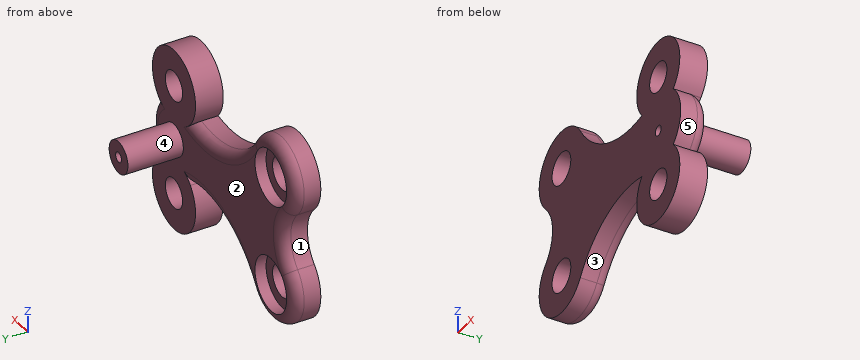
```python
from build123d import *

# Parameters (mm, degrees)
CROQUIS2_R              = 1.45
CROQUIS2_R_2            = 1.335493539
SALIENTE_EXTRUIR1_DEPTH = 2.5
CROQUIS3_R              = 2.45
CORTAR_EXTRUIR1_DEPTH   = 1
CROQUIS4_R              = 1.45
CROQUIS4_R_2            = 0.45
SALIENTE_EXTRUIR2_DEPTH = 5
CROQUIS5_R              = 0.45
CORTAR_EXTRUIR2_DEPTH   = 21.921953183
REDONDEO1_R             = 1


with BuildPart() as part:
    # Croquis2 → Saliente-Extruir1 (new body)
    with BuildSketch(Plane(origin=(0, 0, 0), x_dir=(1, 0, 0), z_dir=(0, 1, 0))):
        with BuildLine():
            ThreePointArc((17.31117806, -2.595010785), (18.475, 0), (17.31117806, 2.595010785))
            ThreePointArc((17.31117806, 2.595010785), (15.166848951, 8.331317844), (12.46008331, 2.837977715))
            ThreePointArc((12.46008331, 2.837977715), (7.057861128, 3.344392229), (2.913938348, 6.8470147))
            ThreePointArc((2.913938348, 6.8470147), (-2.156353419, 7.693072582), (-2.439518395, 2.560481605))
            ThreePointArc((-2.439518395, 2.560481605), (-1.378932188, 0), (-2.439518395, -2.560481605))
            ThreePointArc((-2.439518395, -2.560481605), (-2.156353419, -7.693072582), (2.913938348, -6.8470147))
            ThreePointArc((2.913938348, -6.8470147), (7.057861128, -3.344392229), (12.46008331, -2.837977715))
            ThreePointArc((12.46008331, -2.837977715), (15.166848951, -8.331317844), (17.31117806, -2.595010785))
        make_face()
        with Locations(Location((0, 5, 0), (0, 0, 270))):
            Circle(CROQUIS2_R, mode=Mode.SUBTRACT)
        with Locations(Location((0, -5, 0), (0, 0, 90))):
            Circle(CROQUIS2_R, mode=Mode.SUBTRACT)
        with Locations(Location((15, -5, 0), (0, 0, 270))):
            Circle(CROQUIS2_R_2, mode=Mode.SUBTRACT)
        with Locations(Location((15, 5, 0), (0, 0, 90))):
            Circle(CROQUIS2_R_2, mode=Mode.SUBTRACT)
    extrude(amount=SALIENTE_EXTRUIR1_DEPTH)

    # Croquis3 → Cortar-Extruir1 (cut)
    with BuildSketch(Plane(origin=(0, 2.5, 0), x_dir=(1, 0, 0), z_dir=(0, 1, 0))):
        with Locations(Location((0, 5, 0), (0, 0, 270))):
            Circle(CROQUIS3_R)
        with Locations(Location((0, -5, 0), (0, 0, 270))):
            Circle(CROQUIS3_R)
    extrude(amount=-CORTAR_EXTRUIR1_DEPTH, mode=Mode.SUBTRACT)

    # Croquis4 → Saliente-Extruir2 (add)
    with BuildSketch(Plane(origin=(0, 2.5, 0), x_dir=(1, 0, 0), z_dir=(0, 1, 0))):
        with Locations(Location((15, 0, 0), (0, 0, 270))):
            Circle(CROQUIS4_R)
        with Locations(Location((15, 0, 0), (0, 0, 270))):
            Circle(CROQUIS4_R_2, mode=Mode.SUBTRACT)
    extrude(amount=SALIENTE_EXTRUIR2_DEPTH)

    # Croquis5 → Cortar-Extruir2 (cut, through all)
    with BuildSketch(Plane(origin=(0, 2.5, 0), x_dir=(1, 0, 0), z_dir=(0, 1, 0))):
        with Locations(Location((15, 0, 0), (0, 0, 270))):
            Circle(CROQUIS5_R)
    extrude(amount=-CORTAR_EXTRUIR2_DEPTH, mode=Mode.SUBTRACT)

    # Redondeo1
    # the kernel refuses this fillet: 1 mm, written as the material it takes off along each edge
    with BuildSketch(Plane(origin=(10.565709674, 2.5, 11.697129023), x_dir=(-0.8446198111127597, 0, -0.5353665797151015), z_dir=(-0.5353665797151015, 0, 0.8446198111127597))) as redondeo1_piece_1_section:
        with BuildLine():
            CenterArc((9.059426769 + REDONDEO1_R, REDONDEO1_R), REDONDEO1_R, 180, 90)
            Line((9.059426769, REDONDEO1_R), (9.059426769 - REDONDEO1_R * 0.02, REDONDEO1_R))
            Line((9.059426769 - REDONDEO1_R * 0.02, REDONDEO1_R), (9.059426769 - REDONDEO1_R * 0.02, -REDONDEO1_R * 0.02))
            Line((9.059426769 - REDONDEO1_R * 0.02, -REDONDEO1_R * 0.02), (9.059426769 + REDONDEO1_R, -REDONDEO1_R * 0.02))
            Line((9.059426769 + REDONDEO1_R, -REDONDEO1_R * 0.02), (9.059426769 + REDONDEO1_R, 0))
        make_face()
    redondeo1_piece_1 = revolve(axis=Axis((10.565709674, 2.5, 11.697129023), (0, -1, 0)), revolution_arc=85.516050129, mode=Mode.PRIVATE)
    redondeo1_piece_1 = redondeo1_piece_1 - Plane(origin=(15, 2.217210624, 5), x_dir=(-0.7614815197926343, 0, -0.6481866205147249), z_dir=(0, -1, 0)) * Cylinder(3.335493539, 41, mode=Mode.PRIVATE)
    add(redondeo1_piece_1, mode=Mode.SUBTRACT)
    with BuildSketch(Plane(origin=(15, 2.5, 0), x_dir=(0.007852951460832107, 0, 0.9999691651012815), z_dir=(-0.9999691651012815, 0, 0.007852951460832107))) as redondeo1_piece_2_section:
        with BuildLine():
            CenterArc((3.475 - REDONDEO1_R, -REDONDEO1_R), REDONDEO1_R, 0, 90)
            Line((3.475, -REDONDEO1_R), (3.475 + REDONDEO1_R * 0.02, -REDONDEO1_R))
            Line((3.475 + REDONDEO1_R * 0.02, -REDONDEO1_R), (3.475 + REDONDEO1_R * 0.02, REDONDEO1_R * 0.02))
            Line((3.475 + REDONDEO1_R * 0.02, REDONDEO1_R * 0.02), (3.475 - REDONDEO1_R, REDONDEO1_R * 0.02))
            Line((3.475 - REDONDEO1_R, REDONDEO1_R * 0.02), (3.475 - REDONDEO1_R, 0))
        make_face()
    redondeo1_piece_2 = revolve(axis=Axis((15, 2.5, 0), (0, 1, 0)), revolution_arc=179.1001088, mode=Mode.PRIVATE)
    redondeo1_piece_2 = redondeo1_piece_2 - Plane(origin=(15, 2.215042964, -5), x_dir=(0.6929043732212018, 0, 0.7210294928579091), z_dir=(0, -1, 0)) * Cylinder(3.335493539, 14, mode=Mode.PRIVATE)
    redondeo1_piece_2 = redondeo1_piece_2 - Plane(origin=(15, 2.215042964, 5), x_dir=(-0.7614815197926343, 0, -0.6481866205147249), z_dir=(0, -1, 0)) * Cylinder(3.335493539, 14, mode=Mode.PRIVATE)
    add(redondeo1_piece_2, mode=Mode.SUBTRACT)
    with BuildSketch(Plane(origin=(10.565709674, 2.5, -11.697129023), x_dir=(0.4676957368071937, 0, 0.883889528036381), z_dir=(0.883889528036381, 0, -0.4676957368071937))) as redondeo1_piece_3_section:
        with BuildLine():
            CenterArc((9.059426769 + REDONDEO1_R, REDONDEO1_R), REDONDEO1_R, 180, 90)
            Line((9.059426769 + REDONDEO1_R, 0), (9.059426769 + REDONDEO1_R, -REDONDEO1_R * 0.02))
            Line((9.059426769 + REDONDEO1_R, -REDONDEO1_R * 0.02), (9.059426769 - REDONDEO1_R * 0.02, -REDONDEO1_R * 0.02))
            Line((9.059426769 - REDONDEO1_R * 0.02, -REDONDEO1_R * 0.02), (9.059426769 - REDONDEO1_R * 0.02, REDONDEO1_R))
            Line((9.059426769 - REDONDEO1_R * 0.02, REDONDEO1_R), (9.059426769, REDONDEO1_R))
        make_face()
    redondeo1_piece_3 = revolve(axis=Axis((10.565709674, 2.5, -11.697129023), (0, -1, 0)), revolution_arc=85.516050129, mode=Mode.PRIVATE)
    redondeo1_piece_3 = redondeo1_piece_3 - Plane(origin=(15, 2.217210619, -5), x_dir=(0.6929043732212018, 0, 0.7210294928579091), z_dir=(0, -1, 0)) * Cylinder(3.335493539, 41, mode=Mode.PRIVATE)
    add(redondeo1_piece_3, mode=Mode.SUBTRACT)
    with BuildSketch(Plane(origin=(0, 2.5, -5), x_dir=(0.8446198111127605, 0, -0.5353665797151004), z_dir=(0.5353665797151004, 0, 0.8446198111127605))) as redondeo1_piece_4:
        with BuildLine():
            CenterArc((3.45 - REDONDEO1_R, -REDONDEO1_R), REDONDEO1_R, 0, 90)
            Line((3.45 - REDONDEO1_R, 0), (3.45 - REDONDEO1_R, REDONDEO1_R * 0.02))
            Line((3.45 - REDONDEO1_R, REDONDEO1_R * 0.02), (3.45 + REDONDEO1_R * 0.02, REDONDEO1_R * 0.02))
            Line((3.45 + REDONDEO1_R * 0.02, REDONDEO1_R * 0.02), (3.45 + REDONDEO1_R * 0.02, -REDONDEO1_R))
            Line((3.45 + REDONDEO1_R * 0.02, -REDONDEO1_R), (3.45, -REDONDEO1_R))
        make_face()
    revolve(axis=Axis((0, 2.5, -5), (0, 1, 0)), revolution_arc=192.631224639, mode=Mode.SUBTRACT)
    with BuildSketch(Plane(origin=(-5, 2.5, 0), x_dir=(0.7071067811865475, 0, -0.7071067811865476), z_dir=(-0.7071067811865476, 0, -0.7071067811865475))) as redondeo1_piece_5:
        with BuildLine():
            CenterArc((3.621067812 + REDONDEO1_R, REDONDEO1_R), REDONDEO1_R, 180, 90)
            Line((3.621067812 + REDONDEO1_R, 0), (3.621067812 + REDONDEO1_R, -REDONDEO1_R * 0.02))
            Line((3.621067812 + REDONDEO1_R, -REDONDEO1_R * 0.02), (3.621067812 - REDONDEO1_R * 0.02, -REDONDEO1_R * 0.02))
            Line((3.621067812 - REDONDEO1_R * 0.02, -REDONDEO1_R * 0.02), (3.621067812 - REDONDEO1_R * 0.02, REDONDEO1_R))
            Line((3.621067812 - REDONDEO1_R * 0.02, REDONDEO1_R), (3.621067812, REDONDEO1_R))
        make_face()
    revolve(axis=Axis((-5, 2.5, 0), (0, -1, 0)), revolution_arc=90, mode=Mode.SUBTRACT)
    with BuildSketch(Plane(origin=(0, 2.5, 5), x_dir=(-0.7071067811865475, 0, -0.7071067811865476), z_dir=(0.7071067811865476, 0, -0.7071067811865475))) as redondeo1_piece_6:
        with BuildLine():
            CenterArc((3.45 - REDONDEO1_R, -REDONDEO1_R), REDONDEO1_R, 0, 90)
            Line((3.45, -REDONDEO1_R), (3.45 + REDONDEO1_R * 0.02, -REDONDEO1_R))
            Line((3.45 + REDONDEO1_R * 0.02, -REDONDEO1_R), (3.45 + REDONDEO1_R * 0.02, REDONDEO1_R * 0.02))
            Line((3.45 + REDONDEO1_R * 0.02, REDONDEO1_R * 0.02), (3.45 - REDONDEO1_R, REDONDEO1_R * 0.02))
            Line((3.45 - REDONDEO1_R, REDONDEO1_R * 0.02), (3.45 - REDONDEO1_R, 0))
        make_face()
    revolve(axis=Axis((0, 2.5, 5), (0, 1, 0)), revolution_arc=192.631224639, mode=Mode.SUBTRACT)


solid = part.part
```
CAD build for the part. Positions are in the model's coordinates, mm. Face numbers are marked on the shaded views. A direction names the side the tool comes from. Give positions to 0.01 mm unless a question says otherwise; leave off trailing zeros. Write each loop counter-clockwise with the first axis right and the second up, starting at its lowest first coordinate (ties: lowest second). Pieces come first, ordered by that corner, then holes. Notation, with made-up numbers: M 43,89.25 L 62,89.25 A25 ccw 62,118.25 Z; hole C 59,-10.5 d4. An arc over 180 degrees is marked long. Return JSON: item names as keys, results as strings. Group by question number.
(1) Band-saw the part on C-C (x = 0). Give the cut face in (y, z), and give its area (3 significant figures).
(2) Band-saw the part on D-D (y = 2.25). Give the cut face in (x, z).
(3) Mould opens along X. For the marked faces 1, 2 and 3 say: pulls with the +X half, pulls with the -X half, needs draft (parallel to the pull), parting line crosses it, or undercut.
(4) 3-axis set-ups, long thin cutter, end or side, ignore diameter. For the marked faces 4 and 5: which of +Z, -Z, +X, -X, +Y, -Y reach the whole face in a straight line?
(5) Flat gauge pins, fed straight in: pin 1 Ø8 at (x, z) = (0, -5) entering from +Y; pin 2 Ø1.5 at (x, z) = (3, 6) entering from -Y; pin 3 Ø3 at (y, z) = (1.5, 6.5) entering from +X; pin 4 Ø1.5 at (x, y) = (14, 6) entering from +Z. Where does each tip first touch, or does it go through?
(6) Drill centre lines: L1, parallel to Z at x = 1, y = 1; L2, parallel to X at y = 2, z = 5; L3, parallel to X at y = 0.85, z = 0 (3 decimals). Where is each one in solid material? Low to high. Write a range as [from, to].
(7) Band-saw the part on A-A (x = 15). Give the cut face in (y, z).
(8) Band-saw the part on B-B (z = 0). Give the cut face in (x, y) (3 decimals).
Entries:
{
 "1": {"outline": "M 0,-8.45 L 1.5,-8.45 A1 ccw 2.5,-7.45 L 1.5,-7.45 L 1.5,-6.45 L 0,-6.45 Z; M 0,-3.55 L 1.5,-3.55 L 1.5,-2.55 L 2.5,-2.55 L 2.5,2.55 L 1.5,2.55 L 1.5,3.55 L 0,3.55 Z; M 0,6.45 L 1.5,6.45 L 1.5,7.45 L 2.5,7.45 A1 ccw 1.5,8.45 L 0,8.45 Z", "area": "23.3 mm^2"},
 "2": {"outline": "M -2.2,-2.8 A3.11 ccw long 2.63,-6.67 A9.4 cw 12.73,-2.55 A3.34 ccw long 17.05,-2.37 A3.14 ccw 17.05,2.37 A3.34 ccw long 12.73,2.55 A9.4 cw 2.63,6.67 A3.11 ccw long -2.2,2.8 A3.96 cw Z; hole C 0,-5 d4.9; hole C 0,5 d4.9; hole C 15,-5 d2.67; hole C 15,5 d2.67; hole C 15,0 d0.9"},
 "3": {"face 1": "pulls with the -X half", "face 2": "needs draft", "face 3": "undercut"},
 "4": {"face 4": "+Y", "face 5": "+X, +Y, -Y"},
 "5": {"pin 1": "stops at y = 2.5", "pin 2": "stops at y = 0", "pin 3": "stops at x = 18.34", "pin 4": "stops at z = 1.43"},
 "6": {"L1": "z = [-8.3, -6.05], [-3.95, 3.95], [6.05, 8.3]", "L2": "x = [-3.32, -2.45], [2.45, 4.27], [11.66, 13.66], [16.34, 18.34]", "L3": "x = [-1.379, 14.55], [15.45, 18.475]"},
 "7": {"outline": "M 0,-8.34 L 2.5,-8.34 L 2.5,-6.34 L 0,-6.34 Z; M 0,-3.66 L 2.5,-3.66 L 2.5,-1.45 L 7.5,-1.45 L 7.5,-0.45 L 0,-0.45 Z; M 0,0.45 L 7.5,0.45 L 7.5,1.45 L 2.5,1.45 L 2.5,3.66 L 0,3.66 Z; M 0,6.34 L 2.5,6.34 L 2.5,8.34 L 0,8.34 Z"},
 "8": {"outline": "M -1.379,0 L 14.55,0 L 14.55,7.5 L 13.55,7.5 L 13.55,2.5 L -0.379,2.5 A1 ccw -1.379,1.5 Z; M 15.45,0 L 18.475,0 L 18.475,1.5 A1 ccw 17.475,2.5 L 16.45,2.5 L 16.45,7.5 L 15.45,7.5 Z"}
}
